For this review, take the finished solid that the model builds, in its own axes (mm). Face numbers are marked on the shaded views. A direction names the side the tool comes from. Give positions to 0.01 mm unless a question says otherwise; leave off trailing zeros. Loops run counter-clockwise (first coordinate to the right, second up) from the corner with the lowest first, then second, coordinate; pieces in that order, holes last.
```python
from build123d import *

# Parameters (mm, degrees)
F1_DEPTH = 15
F3_D     = 19.1
F3_DEPTH = 14
F3_TIP   = 5.7382189117
F5_R     = 14.99999
F6_D     = 9.525


# Not quite as in the source:
# - a fillet or chamfer is up to 0.001 mm smaller than in the source, because OpenCascade refuses the exact size
# - a length typed as a fraction of an inch, garbled in the dataset ("3 / 203.2 mm" for 3/8 in), is restored


with BuildPart() as f1:
    # F0 (on Right) → F1 (new body, symmetric)
    with BuildSketch(Plane.YZ):
        Polygon((0, -35), (0, 0), (55, 0), (55, 25), (-25, 25), (-25, 0), (-95, 0), (-95, -25), (-25, -25), (-25, -35), align=None)
    extrude(amount=F1_DEPTH, both=True)

    # F3
    with Locations(Plane(origin=(0, 0, 0), x_dir=(-1, 0, 0), z_dir=(0, 1, 0))):
        with Locations((0, -19.5)):
            Hole(F3_D / 2, depth=F3_DEPTH)
            with Locations((0, 0, -(F3_DEPTH + F3_TIP / 2))):  # 118° drill point
                Cone(0, F3_D / 2, F3_TIP, mode=Mode.SUBTRACT)

    # F5 (radius 15 in the source; OpenCascade refuses exactly that, so slightly less here)
    f5_edges = [f1.edges().sort_by_distance(p)[0] for p in [
        (-15, 55, 12.5),
        (15, 55, 12.5),
    ]]
    fillet(f5_edges, radius=F5_R)

    # F6 (through all)
    with Locations(Plane(origin=(0, 0, 0), x_dir=(1, 0, 0), z_dir=(0, 0, -1))):
        with Locations((0, -39.75)):
            Hole(F6_D / 2)


solid = f1.part
```
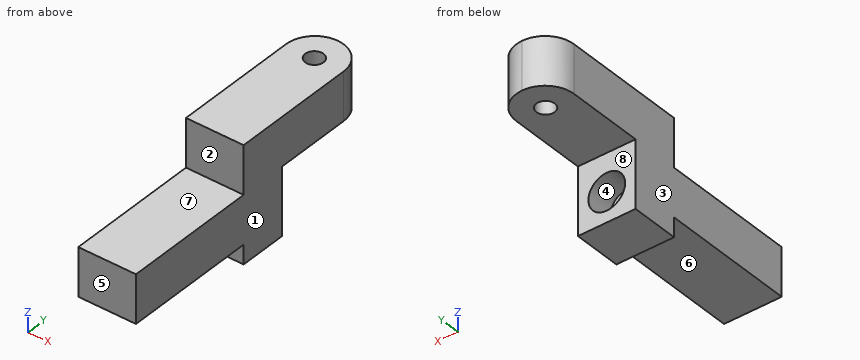
Q1. Mouldability with a two-part tool opening along X and no side actions: class the marked faces 1, 2, 3 and 4 as +X half, -X half, draft (parallel to the pull), parting line (faces both ways), or undercut.
Answers:
face 1: +X half
face 2: draft
face 3: -X half
face 4: undercut
Q2. Machinability: for the marked faces 5, 6, 7 and 8, which of the approach directions +Z, -Z, +X, -X, +Y, -Y give a long, thin tool a straight path to every point of the face, cutting with its end or side? Answer none if there is none.
Answers:
face 5: +Z, -Z, +X, -X, -Y
face 6: -Z, +X, -X, -Y
face 7: +Z, +X, -X, -Y
face 8: -Z, +X, -X, +Y
Q3. For probe 1 along X at (y, z) = (39.75, 12); probe 2 along Z at (x, y) = (0, -10); probe 3 along X at (y, z) = (-7.5, -19.5), list the stretches that pass through material, from the lowest coordinate up.
Answers:
probe 1: x = -15 to -4.76, 4.76 to 15
probe 2: z = -35 to -29.05, -9.95 to 25
probe 3: x = -15 to -9.55, 9.55 to 15
Q4. Consider section B-B on x = 13.5. Give the boundary of the cut face in (y, z), plus the area to 3 significant figures.
Answers:
outline: (-95, -25) - (-25, -25) - (-25, -35) - (0, -35) - (0, 0) - (46.54, 0) - (46.54, 25) - (-25, 25) - (-25, 0) - (-95, 0) - close
area: 4,410 mm2
Q5. Consider section D-D on z = -31. Give the boundary of the cut face in (x, y).
Answers:
outline: (-15, -25) - (15, -25) - (15, 0) - (-15, 0) - close
Q6. Consider section C-C on y = 17. Give the boundary of the cut face in (x, z), plus the area to 3 significant figures.
Answers:
outline: (-15, 0) - (15, 0) - (15, 25) - (-15, 25) - close
area: 750 mm2
Q7. For pin 1 Ø15 at (x, z) = (2, -16.5) entering from +Y; pin 2 Ø9 at (x, y) = (-2, -66.5) entering from -Z; pin 3 Ø2 at (x, z) = (-4.5, -16.5) entering from +Y, all flat-tipped, find the tip position at first contact; note any pin that passes through.
Answers:
pin 1: stops at y = 0
pin 2: stops at z = -25
pin 3: stops at y = -15.89
